```python
from build123d import *

# Parameters (mm, degrees)
SKETCH_W        = 50
SKETCH_H        = 10
PAD_DEPTH       = 3
SKETCH001_W     = 27.748524
SKETCH001_H     = 3.203372
PAD001_DEPTH    = 3
POCKET_DEPTH    = 3.5
FILLET_R        = 1
FILLET001_R     = 1
POCKET001_DEPTH = 0.5


with BuildPart() as part:
    # Sketch → Pad (new body)
    with BuildSketch(Plane.XY):
        Rectangle(SKETCH_W, SKETCH_H)
        with BuildLine():
            ThreePointArc((-21.956885, 1.5), (-23.456885, 0), (-21.956885, -1.5))
            Line((-21.956885, -1.5), (-16.956885, -1.5))
            ThreePointArc((-16.956885, -1.5), (-15.456885, 0), (-16.956885, 1.5))
            Line((-21.956885, 1.5), (-16.956885, 1.5))
        make_face(mode=Mode.SUBTRACT)
        with BuildLine():
            Line((16.956885, 1.5), (21.956885, 1.5))
            ThreePointArc((21.956885, -1.5), (23.456885, 0), (21.956885, 1.5))
            Line((16.956885, -1.5), (21.956885, -1.5))
            ThreePointArc((16.956885, 1.5), (15.456885, 0), (16.956885, -1.5))
        make_face(mode=Mode.SUBTRACT)
    extrude(amount=PAD_DEPTH)

    # Sketch001 (on DatumPlane) → Pad001 (join)
    with BuildSketch(Plane.XY.offset(3)):
        Rectangle(SKETCH001_W, SKETCH001_H)
    extrude(amount=PAD001_DEPTH)

    # Sketch002 (on DatumPlane) → Pocket (cut)
    with BuildSketch(Plane.XZ.offset(1.601686)):
        with BuildLine():
            add(Edge.make_bspline(
                [(-13.874262, 3), (-9.664405, 3.309267), (-11.317866, 5.566879), (-7.216269, 6)],
                knots=[0, 0, 0, 0, 1, 1, 1, 1], degree=3))
            Line((-7.216269, 6), (-7.216269, 6.383823))
            Line((-7.216269, 6.383823), (-14.222651, 6.336395))
            Line((-14.222651, 6.336395), (-14.222651, 3.364603))
            Line((-14.222651, 3.364603), (-13.874262, 3))
        make_face()
    pocket = extrude(amount=-POCKET_DEPTH, mode=Mode.SUBTRACT)

    # Fillet
    fillet_edges = [part.edges().sort_by_distance(p)[0] for p in [
        (3.328997, -1.601686, 6),
    ]]
    fillet(fillet_edges, radius=FILLET_R)

    # Fillet001
    fillet001_edges = [part.edges().sort_by_distance(p)[0] for p in [
        (3.328997, 1.601686, 6),
    ]]
    fillet(fillet001_edges, radius=FILLET001_R)

    # Mirrored: Pocket across Sketch002 V_Axis
    add(pocket.mirror(Plane(origin=(0, -1.601686, 0), x_dir=(0, -1, 0), z_dir=(1, 0, 0))), mode=Mode.SUBTRACT)

    # Sketch003 (on DatumPlane) → Pocket001 (cut)
    with BuildSketch(Plane.XY.offset(3)):
        with BuildLine():
            ThreePointArc((-21.948886, 2.25), (-24.198886, 0), (-21.948886, -2.25))
            Line((-21.948886, -2.25), (-16.996035, -2.25))
            ThreePointArc((-16.996035, -2.25), (-14.746035, 0), (-16.996035, 2.25))
            Line((-21.948886, 2.25), (-16.996035, 2.25))
        make_face()
        with BuildLine():
            ThreePointArc((16.996035, 2.25), (14.746035, 0), (16.996035, -2.25))
            Line((16.996035, -2.25), (22.07169, -2.25))
            ThreePointArc((22.07169, -2.25), (24.32169, 0), (22.07169, 2.25))
            Line((16.996035, 2.25), (22.07169, 2.25))
        make_face()
    extrude(amount=-POCKET001_DEPTH, mode=Mode.SUBTRACT)


solid = part.part
```
Source: CAD feature listing. Evaluate the final solid. Frame: model axes, mm. A direction names the side the tool comes from. Give positions to 0.01 mm unless a question says otherwise; leave off trailing zeros. Order: outer loops, then holes, each group sorted by start corner. A loop starts at its lowest first (then second) coordinate and runs counter-clockwise, first axis right, second up. Notation, with made-up numbers: (23.5, 33.25) -> (77.5, 33.25) arc R4 ccw to (77.5, 39.25) -> close; hole circle Ø2 at (16, -6). An arc over 180 degrees is marked (long way). Use a Markdown table: item, result.
Q1. Pull-direction query (X, two-part tool) for faces 4 (the face through (25, 0, 1)), 5 (the face through (0, -1.602, 4)), 6 (the face through (-20, 2, 2.5)); classes: +X half, -X half, draft (parallel to the pull), parting line (faces both ways), or undercut.
A:
| item | result |
|---|---|
| face 4 | +X half |
| face 5 | draft |
| face 6 | undercut |
Q2. Section A-A (x = 16). Return the cut outline in (y, z), and give its area (3 significant figures).
A:
| item | result |
|---|---|
| outline | (-5, 0) -> (-1.16, 0) -> (-1.16, 2.5) -> (-2.02, 2.5) -> (-2.02, 3) -> (-5, 3) -> close; (1.16, 0) -> (5, 0) -> (5, 3) -> (2.02, 3) -> (2.02, 2.5) -> (1.16, 2.5) -> close |
| area | 22.2 mm^2 |
Q3. Access query for faces 1 (the face through (15.457, 0.033, 1.232)), 2 (the face through (0, 1.602, 4)), 3 (the face through (19, 2, 2.5)). Directions: +Z, -Z, +X, -X, +Y, -Y. A direction counts if a zero-diameter tool reaches every point of the face in a straight line with its end or side. Return the directions, or none.
A:
| item | result |
|---|---|
| face 1 | +Z, -Z |
| face 2 | +Z, +X, -X, +Y |
| face 3 | +Z |
Q4. Material intervals for line 1 (Z direction, x = -21, y = 2); line 2 (Z direction, x = 5.5, y = 4.25); line 3 (X direction, y = -1, z = 5), sorted ascending. Write a range as [from, to].
A:
| item | result |
|---|---|
| line 1 | [0, 2.5] |
| line 2 | [0, 3] |
| line 3 | [-9.95, 9.95] |
Q5. First-contact query: P1, Ø3, axis at x = -19, z = 4, coming from the -Y side; P2, Ø1, axis at x = -3.5, z = 4.5, coming from the +Y side; P3, Ø3, axis at x = -17, y = 0.5, coming from the +Z side; P4, Ø3.5, axis at x = -22, y = 1, coming from the +Z side. Flat tips, straight axial feed; report the tip coordinate or a pass-through.
A:
| item | result |
|---|---|
| P1 | y = -5 |
| P2 | y = 1.6 |
| P3 | z = 2.5 |
| P4 | z = 3 |
Q6. Section B-B (y = 0). State how many separate pieces and enclosed holes the cut face has, and give its area (3 significant figures).
A:
| item | result |
|---|---|
| separate pieces | 3 |
| enclosed holes | 0 |
| area | 163 mm^2 |
Q7. Section C-C (y = -3.5). Return the cut outline in (x, z).
A:
| item | result |
|---|---|
| outline | (-25, 0) -> (25, 0) -> (25, 3) -> (-25, 3) -> close |
